Source: CAD feature listing. Evaluate the final solid. Frame: model axes, mm. Coordinates: 2 decimals unless noted, no trailing zeros. Order: outer loops, then holes, each group sorted by start corner. A loop starts at its lowest first (then second) coordinate and runs counter-clockwise, first axis right, second up.
Autodesk Inventor part; units mm, degrees
ref_plane "YZ Plane" through (0, 0, 0) normal (1, 0, 0) x (0, 1, 0)
ref_plane "XZ Plane" through (0, 0, 0) normal (0, 1, 0) x (-1, 0, 0)
ref_plane "XY Plane" through (0, 0, 0) normal (0, 0, 1) x (1, 0, 0)
sketch "Sketch1" plane through (0, 0, 0) normal (0, 0, 1) x (1, 0, 0)
  circle A0 centre (0, 0) radius 45
  circle A1 centre (0, 0) radius 12
  dimension "d0" = 90
  dimension "d1" = 24
extrude "Extrusion1" add sketch "Sketch1" along normal blind 10
sketch "Sketch2" plane through (0, 0, 10) normal (0, 0, 1) x (1, 0, 0)
  line L0 (27.3, 12.7) -> (40, 12.7)
  line L1 (40, 12.7) -> (40, 0)
  line L2 (40, 0) -> (27.3, 0)
  line L3 (27.3, 0) -> (27.3, 12.7)
  line L4 (40.5, 13.2) -> (26.8, 13.2)
  line L5 (26.8, 13.2) -> (26.8, -0.5)
  line L6 (26.8, -0.5) -> (40.5, -0.5)
  line L7 (40.5, -0.5) -> (40.5, 13.2)
  point P0 (0, 0)
  dimension "d4" = 12.7
  dimension "d5" = 12.7
  dimension "d6" = 40
  dimension "d7" = 0.5
extrude "Extrusion2" cut sketch "Sketch2" against normal blind 6.35 contours L0 L1 L2 L3 | L7 L6 L5 L4
pattern_circular "Circular Pattern1" count 11 over 360 about axis through (0, 0, 0) along (0, 0, 1) of "Extrusion2"
sketch "Sketch3" plane through (0, 0, 10) normal (0, 0, 1) x (1, 0, 0)
  circle A0 centre (20, 0) radius 1.75
  circle A1 centre (14.1421, 14.1421) radius 1.75
  circle A2 centre (0, 20) radius 1.75
  circle A3 centre (-14.1421, 14.1421) radius 1.75
  circle A4 centre (-20, 0) radius 1.75
  circle A5 centre (-14.1421, -14.1421) radius 1.75
  circle A6 centre (0, -20) radius 1.75
  circle A7 centre (14.1421, -14.1421) radius 1.75
  point P0 (0, 0)
  dimension "d13" = 3.5
  dimension "d14" = 20
  dimension "d17" = 360
extrude "Extrusion3" [suppressed]
properties part number "SG01" material "ABS Plastic"
Q1. Pull-direction query (Y, two-part tool) for faces 1 (the flat face through (-32.05, 9.93, 6.87)), 2 (the flat face through (9, -9, 10)); classes: pulls with the +Y half, pulls with the -Y half, needs draft (parallel to the pull), parting line crosses it, or undercut.
Solutions:
face 1: undercut
face 2: needs draft
Q2. Section query C-C on x = -23.5. Output: boundary loops of the cut face in (y, z), plus the area to 3 significant figures.
Solutions:
outline: (-38.38, 0) - (38.38, 0) - (38.38, 10) - (27.88, 10) - (27.88, 3.65) - (15.1, 3.65) - (15.1, 10) - (-15.09, 10) - (-15.09, 3.65) - (-20.66, 3.65) - (-20.66, 10) - (-26.36, 10) - (-26.36, 3.65) - (-33.23, 3.65) - (-33.23, 10) - (-38.38, 10) - close
area: 607 mm2
Q3. Section query B-B on x = 36. Output: boundary loops of the cut face in (y, z), plus the area to 3 significant figures.
Solutions:
outline: (-27, 0) - (27, 0) - (27, 10) - (13.2, 10) - (13.2, 3.65) - (-0.5, 3.65) - (-0.5, 10) - (-7.44, 10) - (-7.44, 3.65) - (-18.89, 3.65) - (-18.89, 10) - (-27, 10) - close
area: 380 mm2
Q4. Material intervals for line 1 along Y through (x, z) = (0, 3); line 2 along X through (y, z) = (-25.5, 9.5); line 3 along Y through (x, z) = (-21.5, 7.5), sorted ascending.
Solutions:
line 1: y = -45 to -12, 12 to 45
line 2: x = -37.08 to -22.76, -11.5 to 11.1, 26.16 to 37.08
line 3: y = -39.53 to -34.96, -24.05 to 16.83, 25.58 to 39.53
Q5. Section query A-A on z = 5.5. Give the number of separate pieces and of enclosed holes in the cut face, plus the area to 3 significant figures.
Solutions:
separate pieces: 1
enclosed holes: 12
area: 3,840 mm2
Q6. Pin query (flat end, axial travel): P1, Ø21.5, axis at x = -19, y = -30, coming from the +Z side; P2, Ø1.5, axis at x = 31.5, z = 8, coming from the -Y side; P3, Ø1, axis at y = 18.5, z = 6, coming from the -X side; P4, Ø1.9, axis at x = 37, z = 7.5, coming from the -Y side. Return the tip coordinate at first contact, or that it passes through.
Solutions:
P1: stops at z = 10
P2: stops at y = -32.85
P3: stops at x = -41.24
P4: stops at y = -26.93
